Check sheet for the drawn part. Datum: minimum x, y, z corner. Units: mm. A direction names the side the tool comes from. Coordinates: 2 decimals unless noted, no trailing zeros. Write each loop counter-clockwise with the first axis right and the second up, starting at its lowest first coordinate (ties: lowest second). Pieces come first, ordered by that corner, then holes. Notation, with made-up numbers: (60.5, 54) - (70.5, 54) arc R18 ccw to (70.5, 70) - close; hole circle Ø10 at (79.25, 83.25). An arc over 180 degrees is marked (long way). Write each question's results on one line, items separated by ' | '.
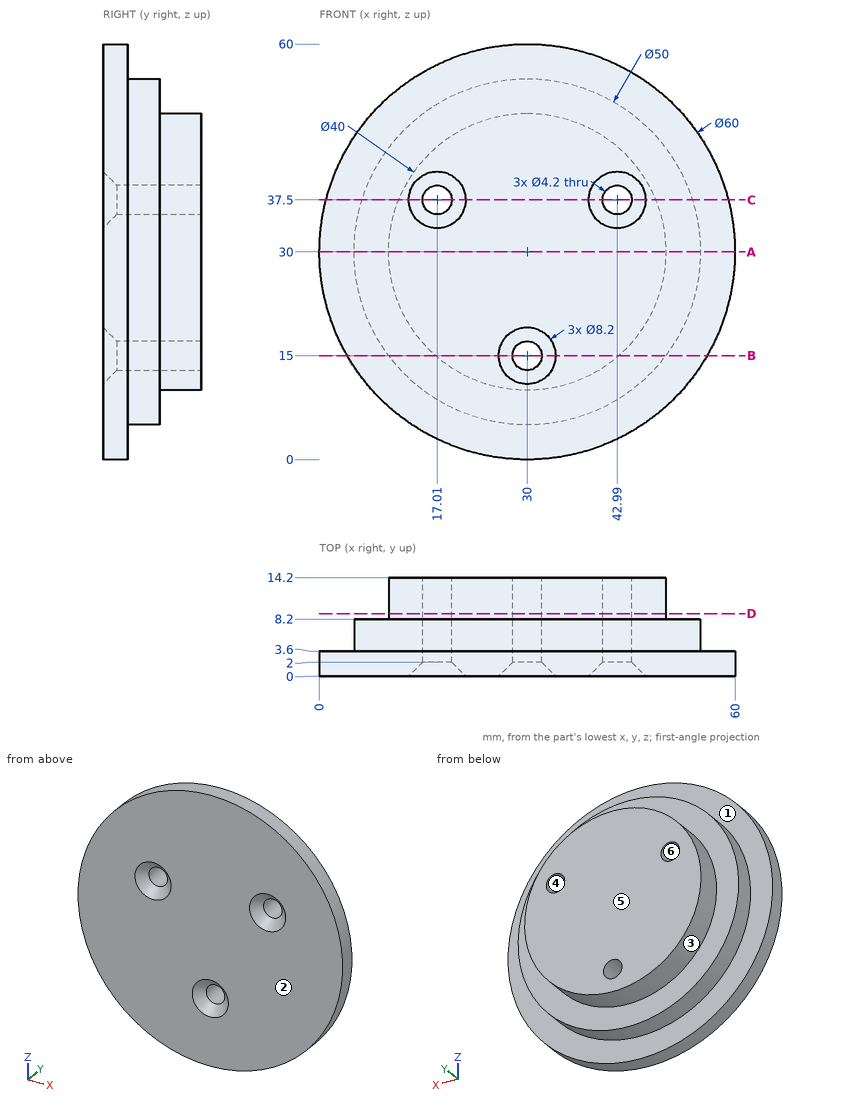
1. Sectioned sample at A-A (z = 30). Record the cut outline in (x, y), then the cut area to 3 significant figures.
Values follow:
outline: (0, 0) - (60, 0) - (60, 3.6) - (55, 3.6) - (55, 8.2) - (50, 8.2) - (50, 14.2) - (10, 14.2) - (10, 8.2) - (5, 8.2) - (5, 3.6) - (0, 3.6) - close | area: 686 mm^2
2. Sectioned sample at B-B (z = 15). Record the cut outline in (x, y).
Values follow:
outline: (4.02, 0) - (25.9, 0) - (27.9, 2) - (27.9, 14.2) - (16.77, 14.2) - (16.77, 8.2) - (10, 8.2) - (10, 3.6) - (4.02, 3.6) - close; (32.1, 2) - (34.1, 0) - (55.98, 0) - (55.98, 3.6) - (50, 3.6) - (50, 8.2) - (43.23, 8.2) - (43.23, 14.2) - (32.1, 14.2) - close
3. Draft check along Z on the marked faces 3, 4, 5 and 6. Enter one of: pulls with the +Z half, pulls with the -Z half, needs draft (parallel to the pull), parting line crosses it, or undercut.
Values follow:
face 3: parting line crosses it | face 4: undercut | face 5: needs draft | face 6: undercut
4. Sectioned sample at D-D (y = 9). Record the cut outline in (x, z), then the cut area to 4 significant figures.
Values follow:
outline: circle Ø40 at (30, 30); hole circle Ø4.2 at (17.01, 37.5); hole circle Ø4.2 at (30, 15); hole circle Ø4.2 at (42.99, 37.5) | area: 1,215 mm^2
5. Sectioned sample at C-C (z = 37.5). Record the cut outline in (x, y).
Values follow:
outline: (0.95, 0) - (12.91, 0) - (14.91, 2) - (14.91, 14.2) - (11.46, 14.2) - (11.46, 8.2) - (6.15, 8.2) - (6.15, 3.6) - (0.95, 3.6) - close; (19.11, 2) - (21.11, 0) - (38.89, 0) - (40.89, 2) - (40.89, 14.2) - (19.11, 14.2) - close; (45.09, 2) - (47.09, 0) - (59.05, 0) - (59.05, 3.6) - (53.85, 3.6) - (53.85, 8.2) - (48.54, 8.2) - (48.54, 14.2) - (45.09, 14.2) - close
6. Material ranges on L1, parallel to X at y = 5, z = 15; L2, parallel to X at y = 8.75, z = 37.5; L3, parallel to Y at x = 40.5, z = 56.5, recorded low to high. Write a range as [from, to].
Values follow:
L1: x = [10, 27.9], [32.1, 50] | L2: x = [11.46, 14.91], [19.11, 40.89], [45.09, 48.54] | L3: y = [0, 3.6]
7. Go/stop test with flat-tipped pins: pin 1 (3 mm diameter, centred on x = 16.5, y = 7, fed in from -Z); pin 2 (6.5 mm diameter, centred on x = 17.01, z = 37.5, fed in from +Y); pin 3 (5 mm diameter, centred on x = 19.5, y = 1.5, fed in from +Z); pin 4 (5 mm diameter, centred on y = 11.5, z = 14.5, fed in from +X). Record where each tip stops, or that it passes through.
Values follow:
pin 1: stops at z = 8.07 | pin 2: stops at y = 14.2 | pin 3: stops at z = 58.91 | pin 4: stops at x = 45.2
8. Access from +Z, -Z, +X, -X, +Y, -Y to the whole of each face (thin tool, end or side, straight path). Record for the marked faces 1 and 2.
Values follow:
face 1: +Y | face 2: +Z, -Z, +X, -X, -Y
